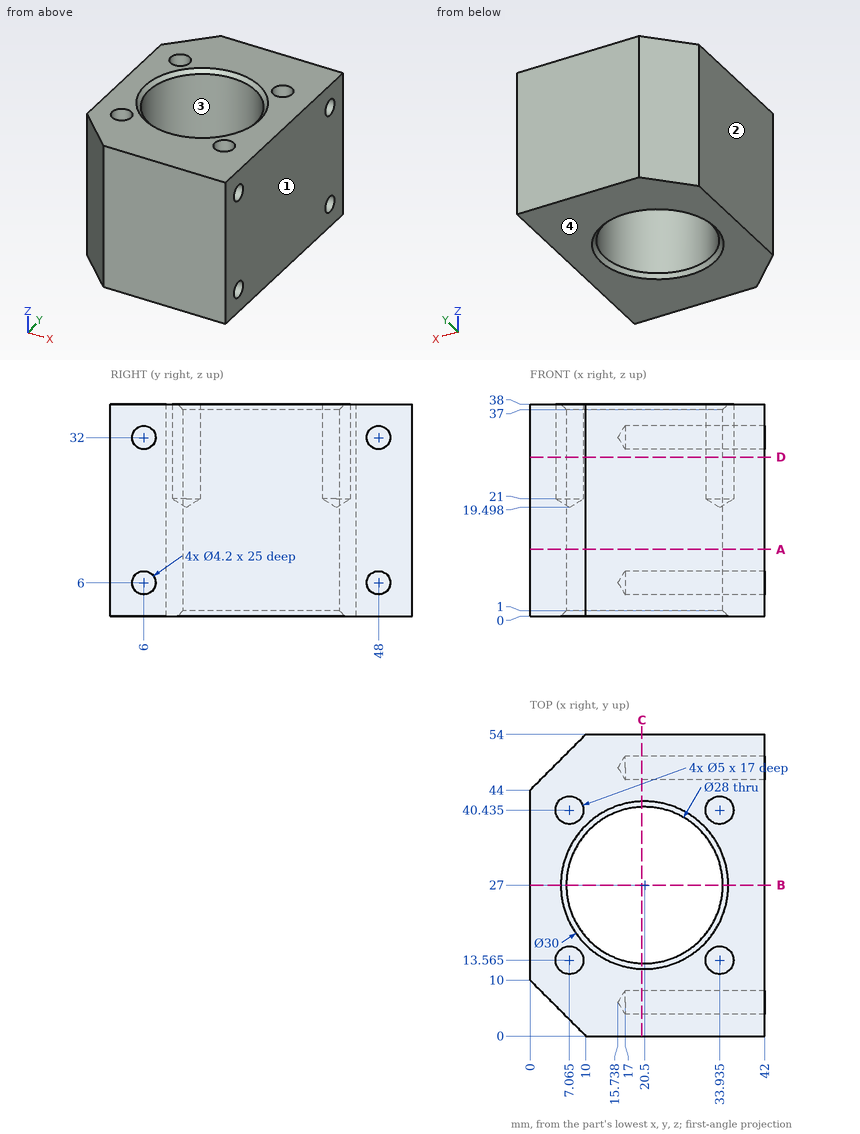
The figure shows three views and two pictorial views of one solid part (mm, origin at its lowest corner). Answer the questions. Round coordinates to 2 decimals unless told otherwise and drop trailing zeros. Loops run counter-clockwise (first coordinate to the right, second up) from the corner with the lowest first, then second, coordinate; pieces in that order, holes last. Notation, with made-up numbers: M 1,-38 L 47,-38 A24 ccw 47,-25 Z; hole C 1.25,65 d6. An arc over 180 degrees is marked long. Use CSV: the item, a comma, the result in double quotes.
Q1. Each of these flat-tipped pins is pushed along its axis until it touches: pin 1 (12 mm diameter, centred on x = 30, y = 22, fed in from -Z); pin 2 (4 mm diameter, centred on y = 48, z = 6, fed in from -X); pin 3 (4 mm diameter, centred on x = 33.94, y = 40.44, fed in from +Z); pin 4 (3.5 mm diameter, centred on y = 6, z = 6, fed in from -X). Where does it stop, or does it pass through?
Determined:
pin 1,"z = 0"
pin 2,"x = 2"
pin 3,"z = 20.7"
pin 4,"x = 2.25"
Q2. Section D-D, the plane z = 28.5 is taken. Determine the outline of the cut face in (x, y) (3 decimals).
Determined:
outline,"M 0,10 L 10,0 L 42,0 L 42,54 L 10,54 L 0,44 Z; hole C 7.065,13.565 d5; hole C 7.065,40.435 d5; hole C 20.5,27 d28; hole C 33.935,13.565 d5; hole C 33.935,40.435 d5"
Q3. Section B-B, the plane y = 27 is taken. Determine the outline of the cut face in (x, z).
Determined:
outline,"M 0,0 L 5.5,0 L 6.5,1 L 6.5,37 L 5.5,38 L 0,38 Z; M 34.5,1 L 35.5,0 L 42,0 L 42,38 L 35.5,38 L 34.5,37 Z"
Q4. Section C-C, the plane x = 20 is taken. State how many separate pieces and enclosed holes the cut face has, then the cut area to 3 significant figures.
Determined:
separate pieces,"2"
enclosed holes,"4"
area,"931 mm2"
Q5. Section A-A, the plane z = 12 is taken. Determine the outline of the cut face in (x, y), then the cut area to 3 significant figures.
Determined:
outline,"M 0,10 L 10,0 L 42,0 L 42,54 L 10,54 L 0,44 Z; hole C 20.5,27 d28"
area,"1,550 mm2"
Q6. The mould has two halves that part along X. Classify the marked faces 1, 2, 3 and 4: pulls with the +X half, pulls with the -X half, needs draft (parallel to the pull), parting line crosses it, or undercut.
Determined:
face 1,"pulls with the +X half"
face 2,"pulls with the -X half"
face 3,"undercut"
face 4,"needs draft"
Q7. Consider L1, parallel to Y at x = 36.5, z = 32; L2, parallel to Z at x = 33.75, y = 6; L3, parallel to Y at x = 20.5, z = 22. Determine where each line is inside the solid, lowest interval first.
Determined:
L1,"0 to 3.9, 8.1 to 45.9, 50.1 to 54"
L2,"0 to 3.9, 8.1 to 29.9, 34.1 to 38"
L3,"0 to 13, 41 to 54"
